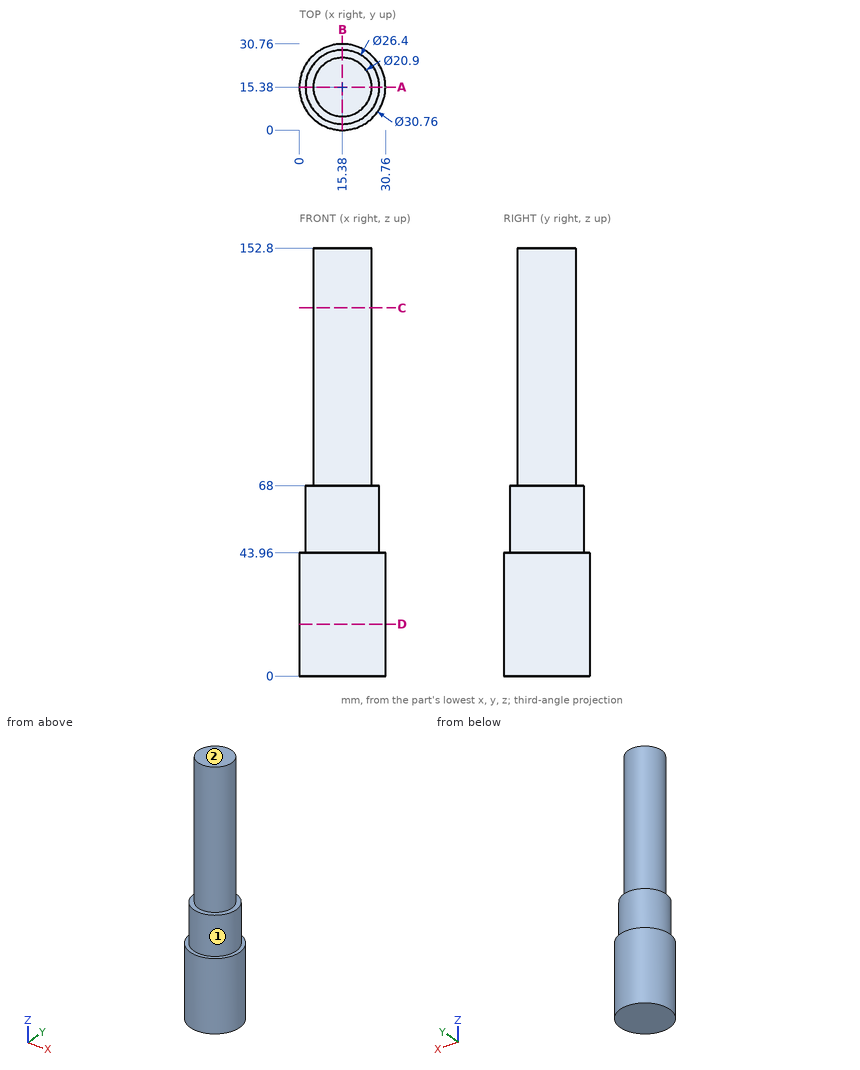
Answer from the drawing. Dimensions are ordinates in mm from the lowest x, y and z of the part. A direction names the side the tool comes from. Give positions to 0.01 mm unless a question says otherwise; leave off trailing zeros. Write each loop counter-clockwise with the first axis right and the second up, starting at its lowest first coordinate (ties: lowest second). Pieces come first, ordered by that corner, then holes. Notation, with made-up numbers: (63, 55) - (96, 55) arc R23 cw to (96, 69) - close; hole circle Ø8 at (35, 68). An arc over 180 degrees is marked (long way). One line per item, written item: value. Start each with the question number.
1. Find section A-A (y = 15.38). Write down the section's boundary in (x, z).
2. Find section D-D (z = 18.5). Write down the section's boundary in (x, y), then the cut area to 3 significant figures.
3. Given pin 1 (8 mm diameter, centred on y = 5.5, z = 69, fed in from +X); pin 2 (1 mm diameter, centred on y = 9, z = 98, fed in from +X); pin 3 (4 mm diameter, centred on x = 6.5, z = 71.5, fed in from +Y), each flat-ended and moving along its own axis, determine where each tip first touches the part or whether it passes through.
4. For the marked faces 1 and 2, determine the directions among +Z, -Z, +X, -X, +Y, -Y from which every point of the face is accessible in a straight line to the end or side of a thin tool.
5. Find section C-C (z = 131.5). Write down the section's boundary in (x, y).
6. Consider probe 1 along X at (y, z) = (16, 129.5); probe 2 along Z at (x, y) = (21, 24.5); probe 3 along Y at (x, z) = (15.5, 21). Determine where each line is inside the solid, lowest interval first.
Geometry results:
1. outline: (0, 0) - (30.76, 0) - (30.76, 43.96) - (28.58, 43.96) - (28.58, 68) - (25.83, 68) - (25.83, 152.8) - (4.93, 152.8) - (4.93, 68) - (2.18, 68) - (2.18, 43.96) - (0, 43.96) - close
2. outline: circle Ø30.76 at (15.38, 15.38)
2. area: 743 mm2
3. pin 1: x = 27.13
3. pin 2: x = 24.02
3. pin 3: y = 23.25
4. face 1: +Z
4. face 2: +Z, +X, -X, +Y, -Y
5. outline: circle Ø20.9 at (15.38, 15.38)
6. probe 1: 4.95 to 25.81
6. probe 2: 0 to 68
6. probe 3: 0 to 30.76
